Verification items for the finished model (mm, model axes). A direction names the side the tool comes from. Coordinates: 2 decimals unless noted, no trailing zeros. Order: outer loops, then holes, each group sorted by start corner. A loop starts at its lowest first (then second) coordinate and runs counter-clockwise, first axis right, second up.
Q1. Depth check by flat-ended pin: P1, Ø5, axis at x = -2.5, y = 47.5, coming from the +Z side; P2, Ø2, axis at x = 37.5, z = 5, coming from the +Y side; P3, Ø10, axis at y = 31.5, z = 24, coming from the +X side; P4, Ø3.5, axis at x = -26, z = 14, coming from the -Y side. Enter the tip coordinate at first touch or a pass-through.
Q2. Draft check along X on faces 1 (the flat face through (37, 23.563, 1)), 2 (the flat face through (1, 49.5, 6)), 3 (the flat face through (56, 61.937, 6)), 4 (the flat face through (-9.5, 23, 6)). Enter one of: pulls with the +X half, pulls with the -X half, needs draft (parallel to the pull), parting line crosses it, or undercut.
Q3. Cross-section at B-B, the plane y = 37. Record the boundary of the cut face in (x, z), and give its area (3 significant figures).
Q4. Set-up check for faces 5 (the flat face through (-14, 17, 10.5)), 6 (the flat face through (-9.5, 16, 23)), 7 (the flat face through (37.498, 4, 14)), 8 (the flat face through (27.04, 24.62, 3.94)): record each of +Z, -Z, +X, -X, +Y, -Y from which the full face is reachable in a straight line by a thin tool's end or side.
Q5. Cross-section at D-D, the plane z = 20.75. Record the boundary of the cut face in (x, y), and give its area (3 significant figures).
Q6. Cross-section at C-C, the plane x = 2. Record the boundary of the cut face in (y, z).
Q7. Thickness scan on line 1 (X direction, y = 1.8, z = 14); line 2 (Y direction, x = 10, z = 7.25); line 3 (Y direction, x = -31, z = 16.75). Record the ranges inside material, lowest first.
Q8. Cross-section at A-A, the plane z = 14. Count the separate pieces of the cut face and the enclosed holes in it, and give its area (3 significant figures).
from build123d import *

# Parameters (mm, degrees)
SKETCH5_R                = 4
BOSS_EXTRUDE1_DEPTH      = 8
SKETCH6_R                = 4
BOSS_EXTRUDE2_DEPTH      = 20
SKETCH7_R                = 7.875
CUT_EXTRUDE1_DEPTH       = 4
SKETCH8_R                = 1.75
CUT_EXTRUDE2_DEPTH       = 64
SKETCH9_R                = 2.25
CUT_EXTRUDE3_DEPTH       = 64
FILLET1_R                = 10
FILLET2_R                = 78
FILLET3_R                = 5
SKETCH10_R               = 11
CUT_EXTRUDE4_DEPTH       = 5
CUT_EXTRUDE5_START       = -5
SKETCH11_R               = 11
CUT_EXTRUDE5_DEPTH       = 5
SKETCH13_R               = 1.75
CUT_EXTRUDE7_DEPTH       = 29
FILLET4_R                = 5
CUT_EXTRUDE8_DEPTH       = 29
CUT_EXTRUDE9_DEPTH       = 3
CUT_EXTRUDE10_START      = -20
SKETCH18_R               = 12.5
CUT_EXTRUDE10_DEPTH      = 20
BOSS_EXTRUDE3_DEPTH      = 3.5
BOSS_EXTRUDE3_DEPTH_BACK = 3.5
SKETCH19_R               = 1.75
CUT_EXTRUDE11_REACH      = 99.703
SKETCH20_W               = 18.5
SKETCH20_H               = 24
SKETCH21_W               = 18.5
SKETCH21_H               = 9.5
CUT_EXTRUDE12_DEPTH      = 5
SKETCH22_W               = 7.5
SKETCH22_H               = 40.5
SKETCH22_W_2             = 10.5
SKETCH22_H_2             = 30.300820781
CUT_EXTRUDE13_DEPTH      = 2
FILLET5_R                = 5
CUT_EXTRUDE14_DEPTH      = 2


with BuildPart() as part:
    # Sketch5 → Boss-Extrude1 (new body)
    with BuildSketch(Plane.XY):
        with BuildLine():
            Line((37.49753719, 0), (-39.50246281, 0))
            Line((-39.50246281, 0), (-39.50246281, 7))
            Line((-39.50246281, 7), (-11.5, 7))
            Line((-11.5, 7), (-11.5, 59))
            Line((-11.5, 59), (29.476702455, 59))
            Line((29.476702455, 59), (53.392166362, 67.704517001))
            ThreePointArc((53.392166362, 67.704517001), (64.120713281, 59.838020936), (52.747381415, 52.936513738))
            ThreePointArc((52.747381415, 52.936513738), (33.77847225, 46.032395426), (40.682590563, 27.063486262))
            ThreePointArc((40.682590563, 27.063486262), (44.048776035, 24.111420832), (45.301644469, 19.813023965))
            ThreePointArc((45.301644469, 19.813023965), (44.871359708, 17.224701884), (43.62679167, 14.91480869))
            Line((43.62679167, 14.91480869), (37.49753719, 7))
            Line((37.49753719, 7), (37.49753719, 0))
        make_face()
        with Locations((3, 35)):
            Circle(SKETCH5_R, mode=Mode.SUBTRACT)
        Polygon((15.5, 7), (15.5, 32), (24.352525767, 32), (33.451781623, 7), align=None, mode=Mode.SUBTRACT)
    extrude(amount=BOSS_EXTRUDE1_DEPTH)

    # Sketch6 → Boss-Extrude2 (add)
    with BuildSketch(Plane.XY.offset(8)):
        Polygon((37.49753719, 0), (-39.50246281, 0), (-39.50246281, 7), (-11.5, 7), (-11.5, 59), (15.5, 59), (15.5, 7), (37.49753719, 7), align=None)
        with Locations((3, 35)):
            Circle(SKETCH6_R, mode=Mode.SUBTRACT)
    extrude(amount=BOSS_EXTRUDE2_DEPTH)

    # Sketch7 → Cut-Extrude1 (cut)
    with BuildSketch(Plane.XZ):
        with Locations(Location((-1.00246281, 14, 0), (0, 0, 270))):
            Circle(SKETCH7_R)
    extrude(amount=-CUT_EXTRUDE1_DEPTH, mode=Mode.SUBTRACT)

    # Sketch8 → Cut-Extrude2 (cut)
    with BuildSketch(Plane(origin=(0, 59, 0), x_dir=(1, 0, 0), z_dir=(0, 1, 0))):
        with Locations(Location((-1.00246281, -14, 0), (0, 0, 180))):
            Circle(SKETCH8_R)
    extrude(amount=-CUT_EXTRUDE2_DEPTH, mode=Mode.SUBTRACT)

    # Sketch9 → Cut-Extrude3 (cut)
    with BuildSketch(Plane.XZ):
        with Locations(Location((23.99753719, 14, 0), (0, 0, 270))):
            Circle(SKETCH9_R)
        with Locations(Location((-26.00246281, 14, 0), (0, 0, 270))):
            Circle(SKETCH9_R)
    extrude(amount=-CUT_EXTRUDE3_DEPTH, mode=Mode.SUBTRACT)

    # Fillet1
    fillet1_edges = [part.edges().sort_by_distance(p)[0] for p in [
        (33.451781623, 7, 4),
    ]]
    fillet(fillet1_edges, radius=FILLET1_R)

    # Fillet2
    fillet2_edges = [part.edges().sort_by_distance(p)[0] for p in [
        (29.476702455, 59, 4),
    ]]
    fillet(fillet2_edges, radius=FILLET2_R)

    # Fillet3
    fillet3_edges = [part.edges().sort_by_distance(p)[0] for p in [
        (15.5, 32, 4),
    ]]
    fillet(fillet3_edges, radius=FILLET3_R)

    # Sketch10 → Cut-Extrude4 (cut)
    with BuildSketch(Plane(origin=(0, 0, 0), x_dir=(-1, 0, 0), z_dir=(0, 0, -1))):
        with Locations((-3, 35)):
            Circle(SKETCH10_R)
    extrude(amount=-CUT_EXTRUDE4_DEPTH, mode=Mode.SUBTRACT)

    # Sketch11 → Cut-Extrude5 (cut)
    with BuildSketch(Plane.XY.offset(28).offset(CUT_EXTRUDE5_START)):
        with Locations(Location((3, 35, 0), (0, 0, 180))):
            Circle(SKETCH11_R)
    extrude(amount=CUT_EXTRUDE5_DEPTH, mode=Mode.SUBTRACT)

    # Sketch13 → Cut-Extrude7 (cut)
    with BuildSketch(Plane.ZY.offset(11.5)):
        with Locations((20.75, 54)):
            Circle(SKETCH13_R)
        with Locations((7.25, 54)):
            Circle(SKETCH13_R)
    extrude(amount=-CUT_EXTRUDE7_DEPTH, mode=Mode.SUBTRACT)

    # Fillet4
    fillet4_edges = [part.edges().sort_by_distance(p)[0] for p in [
        (24.352525767, 32, 4),
    ]]
    fillet(fillet4_edges, radius=FILLET4_R)

    # Sketch14 → Cut-Extrude8 (cut)
    with BuildSketch(Plane.XY.offset(8)):
        with BuildLine():
            Line((58.128327509, 58.436976035), (54.128327509, 58.436976035))
            ThreePointArc((54.128327509, 58.436976035), (52.378327509, 60.186976035), (54.128327509, 61.936976035))
            Line((54.128327509, 61.936976035), (58.128327509, 61.936976035))
            ThreePointArc((58.128327509, 61.936976035), (59.878327509, 60.186976035), (58.128327509, 58.436976035))
        make_face()
        with BuildLine():
            Line((39.301644469, 18.063023965), (35.301644469, 18.063023965))
            ThreePointArc((35.301644469, 18.063023965), (33.551644469, 19.813023965), (35.301644469, 21.563023965))
            Line((35.301644469, 21.563023965), (39.301644469, 21.563023965))
            ThreePointArc((39.301644469, 21.563023965), (41.051644469, 19.813023965), (39.301644469, 18.063023965))
        make_face()
        with BuildLine():
            Line((28.528009954, 47.66334152), (24.528009954, 47.66334152))
            ThreePointArc((24.528009954, 47.66334152), (22.778009954, 49.41334152), (24.528009954, 51.16334152))
            Line((24.528009954, 51.16334152), (28.528009954, 51.16334152))
            ThreePointArc((28.528009954, 51.16334152), (30.278009954, 49.41334152), (28.528009954, 47.66334152))
        make_face()
    extrude(amount=-CUT_EXTRUDE8_DEPTH, mode=Mode.SUBTRACT)

    # Sketch15 → Cut-Extrude9 (cut)
    with BuildSketch(Plane(origin=(0, 0, 0), x_dir=(-1, 0, 0), z_dir=(0, 0, -1))):
        with BuildLine():
            Line((-39.301644469, 16.063023965), (-35.301644469, 16.063023965))
            ThreePointArc((-35.301644469, 16.063023965), (-31.551644469, 19.813023965), (-35.301644469, 23.563023965))
            Line((-35.301644469, 23.563023965), (-39.301644469, 23.563023965))
            ThreePointArc((-39.301644469, 23.563023965), (-43.051644469, 19.813023965), (-39.301644469, 16.063023965))
        make_face()
        with BuildLine():
            Line((-24.528009954, 53.16334152), (-28.528009954, 53.16334152))
            ThreePointArc((-28.528009954, 53.16334152), (-32.278009954, 49.41334152), (-28.528009954, 45.66334152))
            Line((-28.528009954, 45.66334152), (-24.528009954, 45.66334152))
            ThreePointArc((-24.528009954, 45.66334152), (-20.778009954, 49.41334152), (-24.528009954, 53.16334152))
        make_face()
        with BuildLine():
            Line((-54.128327509, 63.936976035), (-58.128327509, 63.936976035))
            ThreePointArc((-58.128327509, 63.936976035), (-61.878327509, 60.186976035), (-58.128327509, 56.436976035))
            Line((-58.128327509, 56.436976035), (-54.128327509, 56.436976035))
            ThreePointArc((-54.128327509, 56.436976035), (-50.378327509, 60.186976035), (-54.128327509, 63.936976035))
        make_face()
    extrude(amount=-CUT_EXTRUDE9_DEPTH, mode=Mode.SUBTRACT)

    # Sketch18 → Cut-Extrude10 (cut)
    with BuildSketch(Plane.XY.offset(28).offset(CUT_EXTRUDE10_START)):
        with Locations((-11.75246281, 35)):
            Circle(SKETCH18_R)
    extrude(amount=CUT_EXTRUDE10_DEPTH, mode=Mode.SUBTRACT)

    # Sketch19 → Boss-Extrude3 (add, two sides: drawn at the far end of the back side and taken through both)
    with BuildSketch(Plane.XY.offset(14).offset(-BOSS_EXTRUDE3_DEPTH_BACK)):
        with BuildLine():
            Line((-19.866362311, 14.172425126), (-11.5, 9))
            Line((-11.5, 9), (-11.5, 22.502549759))
            Line((-11.5, 22.502549759), (-17.501912014, 22.499999594))
            ThreePointArc((-17.501912014, 22.499999594), (-21.828891885, 19.229103353), (-19.866362311, 14.172425126))
        make_face()
        with Locations((-17.5, 18)):
            Circle(SKETCH19_R, mode=Mode.SUBTRACT)
    extrude(amount=BOSS_EXTRUDE3_DEPTH + BOSS_EXTRUDE3_DEPTH_BACK)

    # Cut-Extrude11: up to this face of the body (flat: up to its plane)
    cut_extrude11_end = Plane(part.part.faces().sort_by_distance((-6.507208391, 35, 8))[0])
    # Sketch20 → Cut-Extrude11 (cut, up to the picked face)
    with BuildSketch(Plane.XY.offset(28), mode=Mode.PRIVATE) as cut_extrude11_sk1:
        with Locations((-2.25, 47)):
            Rectangle(SKETCH20_W, SKETCH20_H)
    cut_extrude11_tool1 = split(extrude(cut_extrude11_sk1.sketch, amount=-CUT_EXTRUDE11_REACH, mode=Mode.PRIVATE), bisect_by=cut_extrude11_end, keep=Keep.BOTH, mode=Mode.PRIVATE)
    add(cut_extrude11_tool1.solids().sort_by(Axis((-2.25, 47, 28), (0, 0, -1)))[0], mode=Mode.SUBTRACT)

    # Sketch21 → Cut-Extrude12 (cut)
    with BuildSketch(Plane.XY.offset(8)):
        with Locations((-2.25, 54.25)):
            Rectangle(SKETCH21_W, SKETCH21_H)
    extrude(amount=-CUT_EXTRUDE12_DEPTH, mode=Mode.SUBTRACT)

    # Sketch22 → Cut-Extrude13 (cut)
    with BuildSketch(Plane.ZY.offset(11.5)):
        with Locations((6.75, 29.25)):
            Rectangle(SKETCH22_W, SKETCH22_H)
        with Locations((22.75, 24.150410391)):
            Rectangle(SKETCH22_W_2, SKETCH22_H_2)
    extrude(amount=-CUT_EXTRUDE13_DEPTH, mode=Mode.SUBTRACT)

    # Fillet5
    fillet5_edges = [part.edges().sort_by_distance(p)[0] for p in [
        (-11.5, 59, 1.5),
        (-9.5, 49.5, 5.5),
    ]]
    fillet(fillet5_edges, radius=FILLET5_R)

    # Sketch23 → Cut-Extrude14 (cut)
    with BuildSketch(Plane.XY.offset(8)):
        with BuildLine():
            Line((-9.5, 40), (-8.5, 40))
            ThreePointArc((-8.5, 40), (-3.5, 35), (-8.5, 30))
            Line((-8.5, 30), (-9.5, 30))
            ThreePointArc((-9.5, 30), (-14.5, 35), (-9.5, 40))
        make_face()
    extrude(amount=-CUT_EXTRUDE14_DEPTH, mode=Mode.SUBTRACT)


solid = part.part
Check values:
1. P1: stops at z = 8
1. P2: stops at y = 62.4
1. P3: stops at x = 15.5
1. P4: passes through
2. face 1: undercut
2. face 2: needs draft
2. face 3: undercut
2. face 4: pulls with the -X half
3. outline: (-11.5, 0) - (-7.82, 0) - (-7.82, 5) - (-0.46, 5) - (-0.46, 8) - (-3.92, 8) - (-3.92, 6) - (-9.5, 6) - (-9.5, 3) - (-11.5, 3) - close; (6.46, 5) - (13.82, 5) - (13.82, 0) - (32.76, 0) - (32.76, 8) - (15.5, 8) - (15.5, 28) - (13.82, 28) - (13.82, 23) - (7, 23) - (7, 8) - (6.46, 8) - close
3. area: 340 mm2
4. face 5: -X, +Y
4. face 6: +Z, -X, +Y
4. face 7: +Z, -Z, +X, -Y
4. face 8: +Z, -Z
5. outline: (-39.5, 0) - (-5.06, 0) - (-5.06, 4) - (3.05, 4) - (3.05, 0) - (37.5, 0) - (37.5, 7) - (15.5, 7) - (15.5, 52.25) - (7, 52.25) - (7, 35) arc R4 cw to (0.38, 31.98) arc R12.5 cw to (-9.5, 22.7) - (-9.5, 9) - (-11.5, 9) - (-11.5, 7) - (-39.5, 7) - close; (7, 55.75) - (15.5, 55.75) - (15.5, 59) - (7, 59) - close
5. area: 1,270 mm2
6. outline: (0, 0) - (24.05, 0) - (24.05, 5) - (31.13, 5) - (31.13, 23) - (24.05, 23) - (24.05, 28) - (0, 28) - (0, 21.28) - (4, 21.28) - (4, 6.72) - (0, 6.72) - close; (38.87, 5) - (45.95, 5) - (45.95, 0) - (59, 0) - (59, 3) - (49.5, 3) - (49.5, 8) - (38.87, 8) - close
7. line 1: x = -39.5 to -28.25, -23.75 to -8.88, 6.87 to 21.75, 26.25 to 37.5
7. line 2: y = 0 to 52.25, 55.75 to 59
7. line 3: y = 0 to 7
8. separate pieces: 4
8. enclosed holes: 1
8. area: 1,240 mm2
